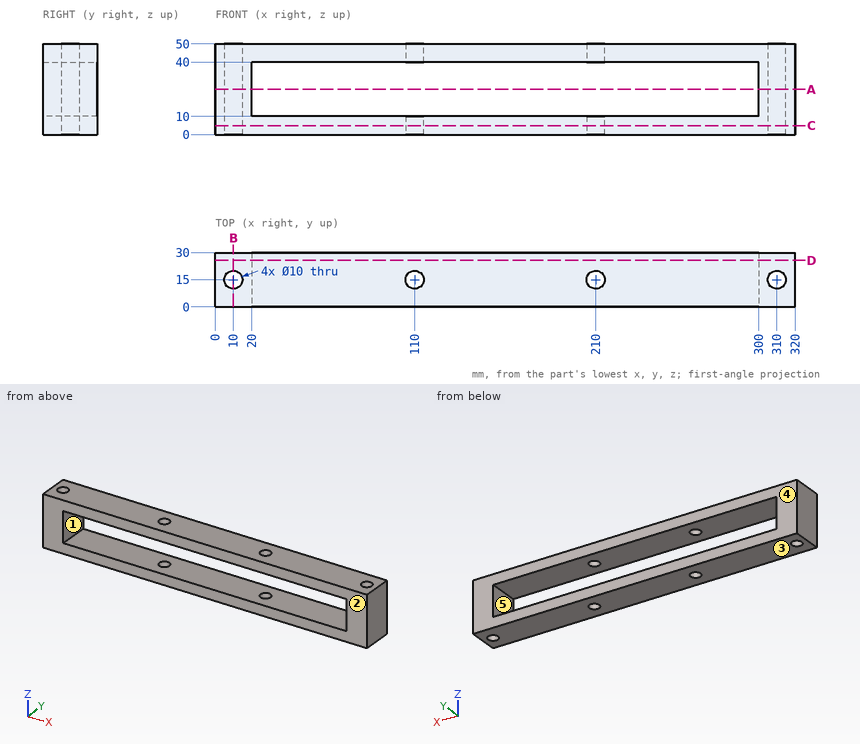
Source: three-view drawing plus pictorial views. Frame: mm from the lowest corner of the part. A direction names the side the tool comes from. Round coordinates to 2 decimals unless told otherwise and drop trailing zeros. Order: outer loops, then holes, each group sorted by start corner. A loop starts at its lowest first (then second) coordinate and runs counter-clockwise, first axis right, second up. Notation, with made-up numbers: M 87,3.5 L 130,3.5 A23 ccw 130,37.5 Z; hole C -13,58 d6. An arc over 180 degrees is marked long. One line per item, written item: value.
(1) Reachability of the marked faces 4 and 5 from +Z, -Z, +X, -X, +Y, -Y: full face, straight path, thin tool, end or side. Return the list, or none.
Result sheet:
face 4: +Z, -Z, +X, -X, +Y
face 5: +Y, -Y
(2) Cut plane B-B (x = 10). Return the cut outline in (y, z).
Result sheet:
outline: M 0,0 L 10,0 L 10,50 L 0,50 Z; M 20,0 L 30,0 L 30,50 L 20,50 Z
(3) Cut plane D-D (y = 25.75). Return the cut outline in (x, z).
Result sheet:
outline: M 0,0 L 320,0 L 320,50 L 0,50 Z; hole M 20,10 L 300,10 L 300,40 L 20,40 Z
(4) Cut plane C-C (z = 5). Return the cut outline in (x, y).
Result sheet:
outline: M 0,0 L 320,0 L 320,30 L 0,30 Z; hole C 10,15 d10; hole C 110,15 d10; hole C 210,15 d10; hole C 310,15 d10
(5) Line query: probe 1 along X at (y, z) = (15, 44.75); probe 2 along Z at (x, y) = (31, 22.25); probe 3 along X at (y, z) = (17.75, 32). Output: solid intervals per line, ascending. Write a range as [from, to].
Result sheet:
probe 1: [0, 5], [15, 105], [115, 205], [215, 305], [315, 320]
probe 2: [0, 10], [40, 50]
probe 3: [0, 5.82], [14.18, 20], [300, 305.82], [314.18, 320]
(6) Cut plane A-A (z = 25). Return the cut outline in (x, y), and give its area (3 significant figures).
Result sheet:
outline: M 0,0 L 20,0 L 20,30 L 0,30 Z; M 300,0 L 320,0 L 320,30 L 300,30 Z; hole C 10,15 d10; hole C 310,15 d10
area: 1,040 mm2
(7) Pull-direction query (Z, two-part tool) for the marked faces 1, 2 and 3; classes: pulls with the +Z half, pulls with the -Z half, needs draft (parallel to the pull), parting line crosses it, or undercut.
Result sheet:
face 1: undercut
face 2: needs draft
face 3: pulls with the -Z half
